The figure shows three views and two pictorial views of one solid part (mm, origin at its lowest corner). Answer the questions. A direction names the side the tool comes from. Coordinates: 2 decimals unless noted, no trailing zeros. Order: outer loops, then holes, each group sorted by start corner. A loop starts at its lowest first (then second) coordinate and runs counter-clockwise, first axis right, second up. Notation, with made-up numbers: (72.25, -4) -> (128.25, -4) arc R25 cw to (128.25, 32) -> close; hole circle Ø8 at (-34, 33). An arc over 180 degrees is marked (long way). Return JSON: item names as keys, results as strings.
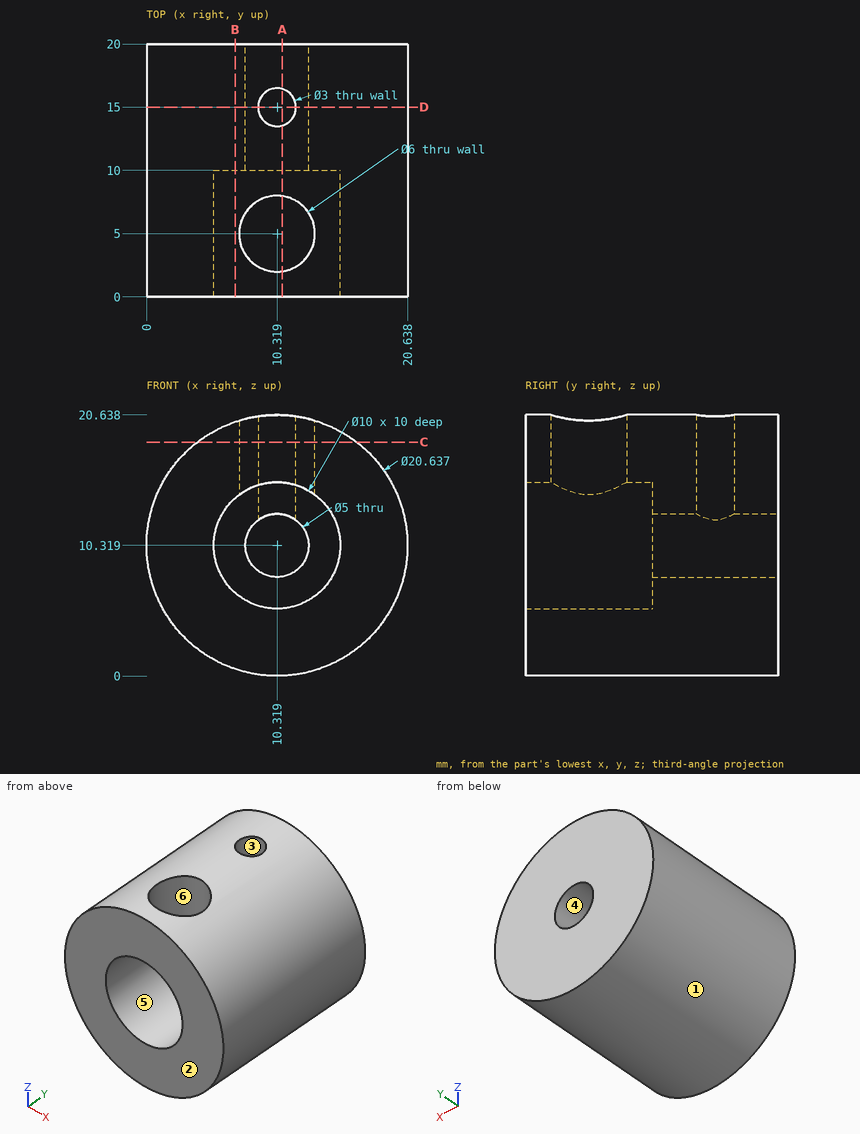
Item 1: Find the intervals of material crossed by probe 1 along Y at (x, z) = (15, 11.5); probe 2 along X at (y, z) = (8.25, 11.25) (1 decimal); probe 3 along Z at (x, y) = (12, 10.5), in increasing order.
Answer list:
{"probe 1": "10 to 20", "probe 2": "0 to 5.4, 15.2 to 20.6", "probe 3": "0.14 to 8.47, 12.17 to 20.5"}
Item 2: Determine the mould class of the marked faces 1, 2 and 3 for opening direction X: pulls with the +X half, pulls with the -X half, needs draft (parallel to the pull), parting line crosses it, or undercut.
Answer list:
{"face 1": "parting line crosses it", "face 2": "needs draft", "face 3": "undercut"}
Item 3: The part is cut by section A-A on x = 10.75. Determine the outline of the cut face in (y, z), plus the area to 3 significant figures.
Answer list:
{"outline": "(0, 0.01) -> (20, 0.01) -> (20, 7.86) -> (10, 7.86) -> (10, 5.34) -> (0, 5.34) -> close; (0, 15.3) -> (2.03, 15.3) -> (2.03, 20.63) -> (0, 20.63) -> close; (7.97, 15.3) -> (10, 15.3) -> (10, 12.78) -> (13.56, 12.78) -> (13.56, 20.63) -> (7.97, 20.63) -> close; (16.44, 12.78) -> (20, 12.78) -> (20, 20.63) -> (16.44, 20.63) -> close", "area": "209 mm2"}
Item 4: The part is cut by section D-D on y = 15. Determine the outline of the cut face in (x, z), plus the area to 3 significant figures.
Answer list:
{"outline": "(8.82, 12.32) -> (8.82, 20.53) arc R10.32 ccw (long way) to (11.82, 20.53) -> (11.82, 12.32) arc R2.5 cw (long way) to start", "area": "291 mm2"}
Item 5: Which of the six approach directions +Z, -Z, +X, -X, +Y, -Y give full straight-line access (tool end or side, diameter ignored) to the marked faces 4, 5 and 6?
Answer list:
{"face 4": "+Y, -Y", "face 5": "-Y", "face 6": "+Z"}
Item 6: The part is cut by section B-B on x = 7. Determine the outline of the cut face in (y, z).
Answer list:
{"outline": "(0, 0.55) -> (20, 0.55) -> (20, 20.09) -> (0, 20.09) -> (0, 14.06) -> (10, 14.06) -> (10, 6.58) -> (0, 6.58) -> close"}
Item 7: The part is cut by section C-C on z = 18.5. Determine the outline of the cut face in (x, y), plus the area to 3 significant figures.
Answer list:
{"outline": "(4.03, 0) -> (16.61, 0) -> (16.61, 20) -> (4.03, 20) -> close; hole circle Ø6 at (10.32, 5); hole circle Ø3 at (10.32, 15)", "area": "216 mm2"}
Item 8: Flat-ended cylindrical pins translate along their axes: pin 1 (3 mm diameter, centred on x = 13, z = 9, fed in from -Y); pin 2 (1 mm diameter, centred on x = 8, y = 3, fed in from -Z); pin 3 (1.5 mm diameter, centred on y = 8.5, z = 5.5, fed in from -X) (1 decimal). Find the tip coordinate at first contact, or state that the pin passes through.
Answer list:
{"pin 1": "y = 10", "pin 2": "z = 0.16", "pin 3": "x = 0.8"}
